Drawing for the job (mm, zero at the part's lowest x, y, z). A direction names the side the tool comes from. Give positions to 0.01 mm unless a question says otherwise; leave off trailing zeros. Order: outer loops, then holes, each group sorted by start corner. A loop starts at its lowest first (then second) coordinate and runs counter-clockwise, first axis right, second up. Notation, with made-up numbers: (0.5, 45) - (10.5, 45) arc R6 cw to (10.5, 49) - close; hole circle Ø1 at (68.25, -13.75). An arc over 180 degrees is marked (long way). Use a Markdown table: item, result. Add a question column.
(1) Slice it at B-B (z = 6). Write the cut outline in (x, y), then the cut area to 3 significant figures.
(2) Slice it at D-D (y = 1.95). Write the cut outline in (x, z) (3 decimals).
(3) Wall check: line 1 (Y direction, x = 9, z = 5.5); line 2 (X direction, y = 8, z = 5.5); line 3 (X direction, y = 1, z = 3.25). Give the ranges that are in metal, low to high.
(4) Slice it at A-A (z = 7.5). Write the cut outline in (x, y).
(5) Flat gauge pins, fed straight in: pin 1 (2 mm diameter, centred on x = 4.74, y = 1.93, fed in from -Z) (3 decimals); pin 2 (1.5 mm diameter, centred on x = 8.5, y = 4, fed in from -Z) (3 decimals); pin 3 (1.5 mm diameter, centred on y = 1.95, z = 5.475, fed in from -X) (3 decimals). Where does each tip first touch, or does it go through?
(6) Slice it at C-C (x = 6.5). Write the cut outline in (y, z).
(7) Which spindle directions (+Z, -Z, +X, -X, +Y, -Y) get a long thin tool onto all of the face, cutting with end or side? Do the marked faces 1 and 2. Say none if no direction does.
(8) Mould opens along X. For the marked faces 3, 4, 5 and 6 say: +X half, -X half, draft (parallel to the pull), parting line (faces both ways), or undercut.
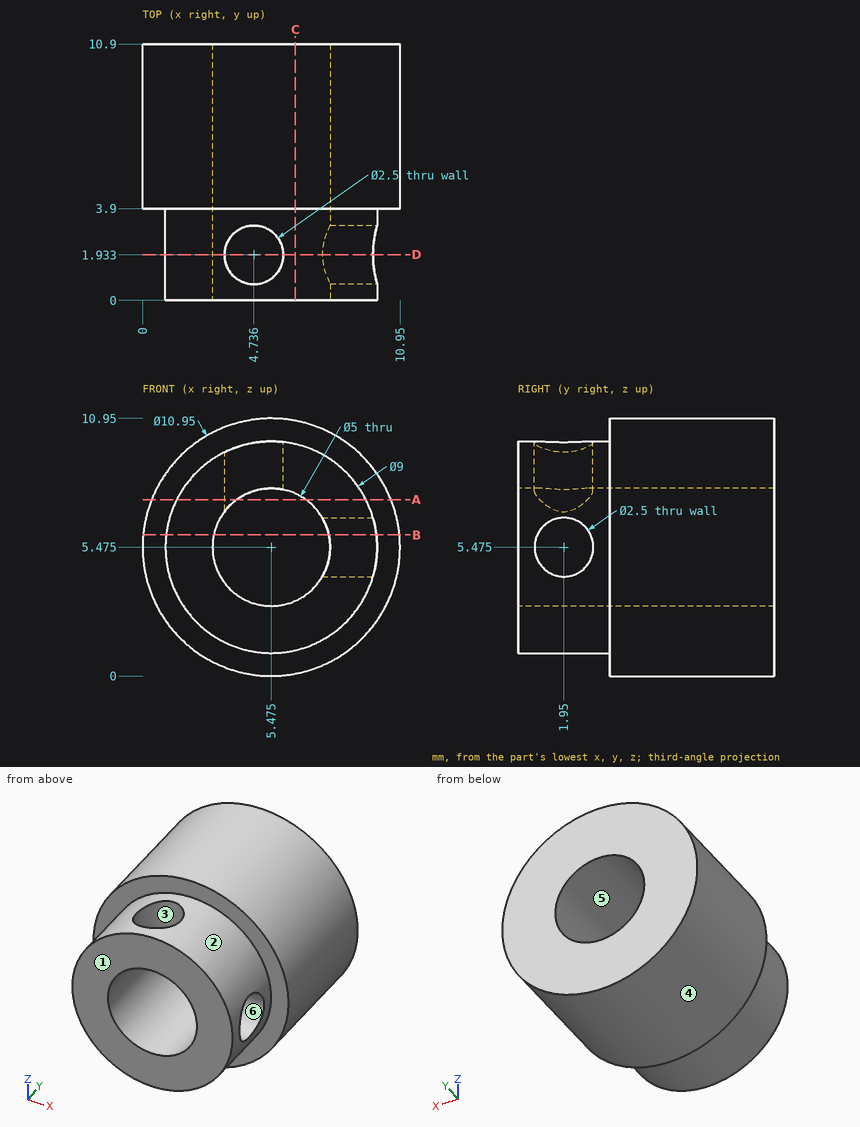
Solution:
| question | item | result |
|---|---|---|
| 1 | outline | (0.03, 3.9) - (1.01, 3.9) - (1.01, 0) - (3.03, 0) - (3.03, 10.9) - (0.03, 10.9) - close; (7.92, 0) - (9.94, 0) - (9.94, 0.82) - (7.92, 0.82) - close; (7.92, 3.08) - (9.94, 3.08) - (9.94, 3.9) - (10.92, 3.9) - (10.92, 10.9) - (7.92, 10.9) - close |
| 1 | area | 53.3 mm2 |
| 2 | outline | (3.486, 6.99) - (3.486, 9.512) arc R4.5 ccw (long way) to (9.798, 4.225) - (7.64, 4.225) arc R2.5 cw (long way) to start; (5.986, 7.922) arc R2.5 cw to (7.64, 6.725) - (9.798, 6.725) arc R4.5 ccw to (5.986, 9.946) - close |
| 3 | line 1 | 0 to 0.7, 3.2 to 10.9 |
| 3 | line 2 | 0 to 2.98, 7.97 to 10.95 |
| 3 | line 3 | 1.56 to 4.34, 6.61 to 9.39 |
| 4 | outline | (0.39, 3.9) - (1.46, 3.9) - (1.46, 0) - (4.01, 0) - (4.01, 0.92) arc R1.25 cw to (4.01, 2.95) - (4.01, 10.9) - (0.39, 10.9) - close; (6.94, 0) - (9.49, 0) - (9.49, 3.9) - (10.56, 3.9) - (10.56, 10.9) - (6.94, 10.9) - close |
| 5 | pin 1 | z = 0.975 |
| 5 | pin 2 | z = 0.495 |
| 5 | pin 3 | x = 0.975 |
| 6 | outline | (0, 1.09) - (3.9, 1.09) - (3.9, 0.1) - (10.9, 0.1) - (10.9, 3.19) - (0, 3.19) - close; (0, 7.76) - (10.9, 7.76) - (10.9, 10.85) - (3.9, 10.85) - (3.9, 9.86) - (0, 9.86) - close |
| 7 | face 1 | +Z, -Z, +X, -X, -Y |
| 7 | face 2 | -Y |
| 8 | face 3 | undercut |
| 8 | face 4 | parting line |
| 8 | face 5 | undercut |
| 8 | face 6 | draft |
